from build123d import *

# Parameters (mm, degrees)
SKETCH_1_W          = 66
SKETCH_1_H          = 23
SKETCH_1_R          = 2
SKETCH_1_R_2        = 1.5
EXTRUDE_1_DEPTH     = 3
CUT_EXTRUDE_1_DEPTH = 46.311168738


with BuildPart() as part:
    # 草图1 → 凸台-拉伸1 (new body)
    with BuildSketch(Plane.XY):
        with Locations((4.349837666, 13.977276909)):
            Rectangle(SKETCH_1_W, SKETCH_1_H)
        with Locations((-5.650162334, 21.977276909)):
            Circle(SKETCH_1_R, mode=Mode.SUBTRACT)
        with Locations((-25.650162334, 21.977276909)):
            Circle(SKETCH_1_R, mode=Mode.SUBTRACT)
        with Locations(Location((14.349837666, 21.977276909, 0), (0, 0, 180))):
            Circle(SKETCH_1_R, mode=Mode.SUBTRACT)
        with Locations(Location((34.349837666, 21.977276909, 0), (0, 0, 180))):
            Circle(SKETCH_1_R, mode=Mode.SUBTRACT)
        with Locations((34.349837666, 17.477276909)):
            Circle(SKETCH_1_R, mode=Mode.SUBTRACT)
        with Locations((14.349837666, 17.477276909)):
            Circle(SKETCH_1_R, mode=Mode.SUBTRACT)
        with Locations(Location((-5.650162334, 17.477276909, 0), (0, 0, 180))):
            Circle(SKETCH_1_R, mode=Mode.SUBTRACT)
        with Locations(Location((-25.650162334, 17.477276909, 0), (0, 0, 180))):
            Circle(SKETCH_1_R, mode=Mode.SUBTRACT)
        with Locations((-8.150162334, 5.977276909)):
            Circle(SKETCH_1_R_2, mode=Mode.SUBTRACT)
        with Locations(Location((16.849837666, 5.977276909, 0), (0, 0, 180))):
            Circle(SKETCH_1_R_2, mode=Mode.SUBTRACT)
    extrude(amount=EXTRUDE_1_DEPTH)

    # 草图2 → 切除-拉伸1 (cut, through all)
    with BuildSketch(Plane.XY.offset(3)):
        Polygon((-28.650162334, 11.707841664), (-19.517537848, 11.707841664), (-11.650162334, 2.477276909), (-28.650162334, 2.477276909), align=None)
        Polygon((20.349837666, 2.477276909), (37.349837666, 2.477276909), (37.349837666, 11.707841664), (28.217213181, 11.707841664), align=None)
    extrude(amount=-CUT_EXTRUDE_1_DEPTH, mode=Mode.SUBTRACT)


solid = part.part
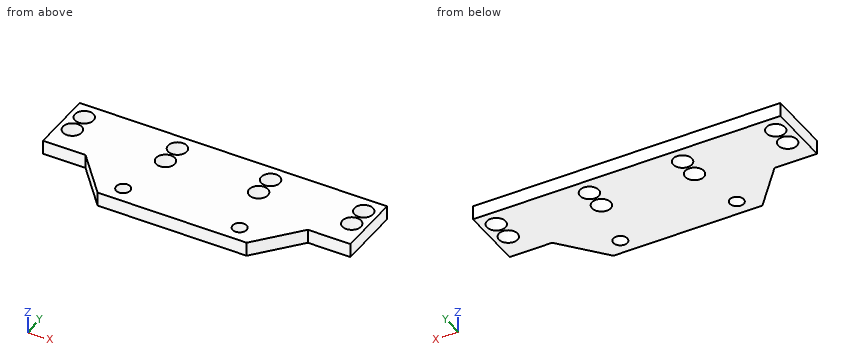
Input: part model. Units: mm. Frame: model coordinates. Coordinates: 2 decimals unless noted, no trailing zeros. Write each loop counter-clockwise with the first axis right and the second up, starting at its lowest first coordinate (ties: lowest second). Pieces come first, ordered by that corner, then holes. Notation, with made-up numbers: M -22.5,69.25 L 27.5,69.25 A34 ccw 27.5,105.25 Z; hole C -14,35.5 d8. An arc over 180 degrees is marked long. Answer as a JSON object with one key per item and string values. Group by question number.
(1) Section C-C on x = -22.5. Output: boundary loops of the cut face in (y, z), plus the area to 3 significant figures.
(2) Section D-D on y = 11. Output: boundary loops of the cut face in (x, z), plus the area to 3 significant figures.
(3) Section A-A on y = 23.25. Output: boundary loops of the cut face in (x, z), plus the area to 3 significant figures.
(4) Contact query for a flat-ended pin moving along its axis: P1, Ø0.9, axis at x = 31, z = 2, coming from the -Y side. Output: stop coordinate, or through.
(5) Section B-B on z = 1.35. Give the number of separate pieces and of enclosed holes in the cut face, plus the area to 3 significant figures.
(6) Ray query, line 1 along Y through (x, z) = (17, 2.7); line 2 along X through (y, z) = (17.25, 0.9); line 3 along X through (y, z) = (6.5, 0.4). Return the intervals inside material, ascending. Write a range as [from, to].
Result set:
{
 "1": {"outline": "M 11.71,0 L 25.48,0 L 25.48,3 L 11.71,3 Z", "area": "41.3 mm2"},
 "2": {"outline": "M -18.91,0 L 27.61,0 L 27.61,3 L -18.91,3 Z", "area": "140 mm2"},
 "3": {"outline": "M -28.65,0 L -27.19,0 L -27.19,3 L -28.65,3 Z; M -24.11,0 L -7.19,0 L -7.19,3 L -24.11,3 Z; M -4.11,0 L 12.81,0 L 12.81,3 L -4.11,3 Z; M 15.89,0 L 32.81,0 L 32.81,3 L 15.89,3 Z; M 35.89,0 L 37.35,0 L 37.35,3 L 35.89,3 Z", "area": "161 mm2"},
 "4": {"P1": "stops at y = 11.71"},
 "5": {"separate pieces": "1", "enclosed holes": "10", "area": "1,160 mm2"},
 "6": {"line 1": "y = [2.48, 4.48], [7.47, 25.48]", "line 2": "x = [-28.65, -27.64], [-23.66, -7.64], [-3.66, 12.36], [16.34, 32.36], [36.34, 37.35]", "line 3": "x = [-15.08, -9.56], [-6.74, 15.44], [18.26, 23.78]"}
}
